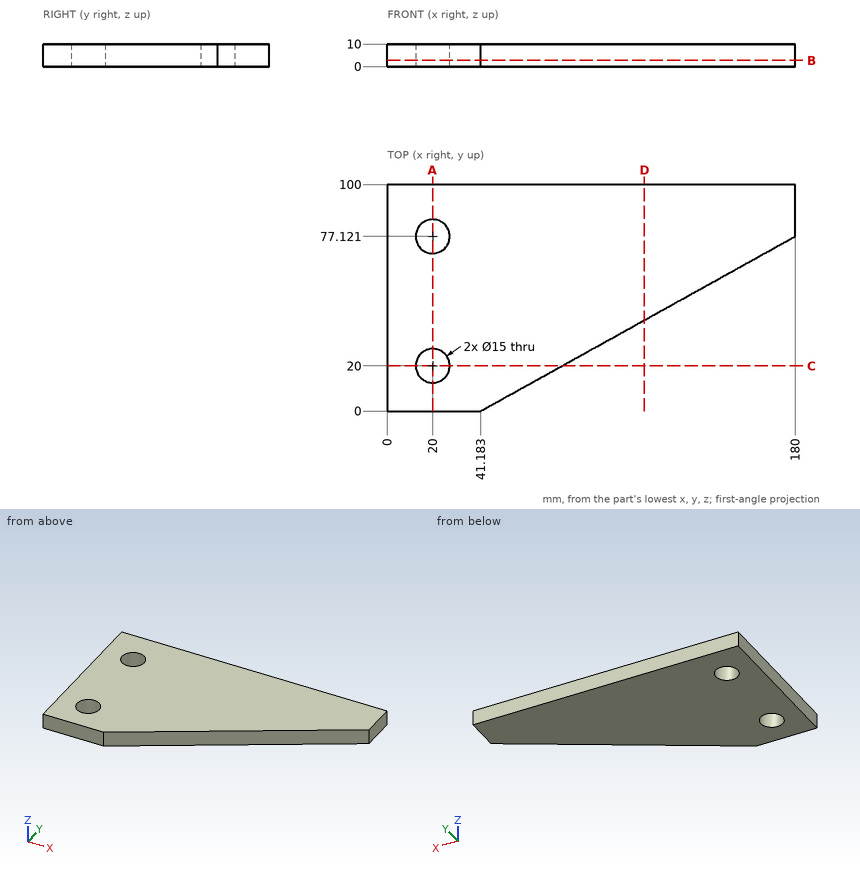
Geometry check sheet. Reference: drawing and pictorial views, mm from the part's lowest x, y, z. Give positions to 0.01 mm unless a question says otherwise; leave off trailing zeros. Order: outer loops, then holes, each group sorted by start corner. A loop starts at its lowest first (then second) coordinate and runs counter-clockwise, first axis right, second up. Notation, with made-up numbers: (5, 20) -> (17, 20) arc R29 cw to (17, 42) -> close; hole circle Ø3 at (-20.75, 18.25). An arc over 180 degrees is marked (long way). Write each question's results on one line, items separated by ' | '. Start each with the question number.
(1) Sectioned sample at A-A (x = 20). Enter the section's corners in (y, z).
(2) Sectioned sample at B-B (z = 2.75). Enter the section's corners in (x, y), plus the area to 3 significant figures.
(3) Gauge pin test, flat end, axial feed: P1, Ø3, axis at x = 129.5, z = 3, coming from the -Y side. Record the tip position at first contact, or that the pin passes through.
(4) Sectioned sample at D-D (x = 113.5). Enter the section's corners in (y, z).
(5) Scan lines: line 1 (Y direction, x = 20, z = 5.75); line 2 (X direction, y = 81, z = 3); line 3 (X direction, y = 6, z = 4.25) (1 decimal). Record each from-to range of solid material in increasing order.
(6) Sectioned sample at C-C (y = 20). Enter the section's corners in (x, z), plus the area to 3 significant figures.
Answer below:
1) outline: (0, 0) -> (12.5, 0) -> (12.5, 10) -> (0, 10) -> close; (27.5, 0) -> (69.62, 0) -> (69.62, 10) -> (27.5, 10) -> close; (84.62, 0) -> (100, 0) -> (100, 10) -> (84.62, 10) -> close
2) outline: (0, 0) -> (41.18, 0) -> (180, 77.12) -> (180, 100) -> (0, 100) -> close; hole circle Ø15 at (20, 20); hole circle Ø15 at (20, 77.12) | area: 12,300 mm2
3) P1: y = 48.23
4) outline: (40.18, 0) -> (100, 0) -> (100, 10) -> (40.18, 10) -> close
5) line 1: 0 to 12.5, 27.5 to 69.62, 84.62 to 100 | line 2: 0 to 13.58, 26.42 to 180 | line 3: 0 to 52
6) outline: (0, 0) -> (12.5, 0) -> (12.5, 10) -> (0, 10) -> close; (27.5, 0) -> (77.18, 0) -> (77.18, 10) -> (27.5, 10) -> close | area: 622 mm2
